Here's how the part is built. I have some questions about the finished solid (model axes, mm). A direction names the side the tool comes from. Coordinates: 2 decimals unless noted, no trailing zeros. Write each loop counter-clockwise with the first axis right and the second up, starting at its lowest first coordinate (ties: lowest second). Pieces come first, ordered by that corner, then holes.
Item 1: For faces 1 (the face through (-10.662, -17, 3)), 2 (the face through (-0.515, -38.635, 0.601)), which set-ups out of +Z, -Z, +X, -X, +Y, -Y let a thin tool reach every point of the face, with its end or its side?
Item 2: If we section it at A-A (z = 3.9): Please give me the cut outline in (x, y), then the cut area to 3 significant figures.
Item 3: If we section it at B-B (x = 8.75): Please give me the cut outline in (y, z), then the cut area to 3 significant figures.
Item 4: I'm going to push a flat-ended pin straight in: pin 1 Ø5 at (x, y) = (3.5, -13) entering from +Z. Where does the tip first touch, or does it pass through?
Item 5: We'd pull the mould along X, two halves only. Please class faces 3 (the face through (-1, -36.706, 3)), 4 (the face through (-12.59, -16.42, 0.6)), 5 (the face through (-1, -39.206, 4)): +X half, -X half, draft (parallel to the pull), parting line (faces both ways), or undercut.
Item 6: If I drill on line 1 (Y direction, x = -3.5, z = 2.65); line 2 (X direction, y = -20, z = 3.55); line 3 (Z direction, x = -2.75, y = -17), over which ranges is the centre line in solid material (lowest first)?
Item 7: If we section it at C-C (y = -21.5): Please give me the cut outline in (x, z).
from build123d import *

# Parameters (mm, degrees)
IZIM1_W                     = 25
IZIM1_H                     = 45
Y_KSEKLIK_EKSTR_ZYON1_DEPTH = 5
IZIM2_W                     = 20
IZIM2_H                     = 40
KES_EKSTR_ZYON1_DEPTH       = 3.5
RADYUS1_R                   = 2


with BuildPart() as part:
    # Çizim1 → Yükseklik-Ekstrüzyon1 (new body)
    with BuildSketch(Plane.XY.offset(5)):
        with Locations((-0.661993769, -16.705607477)):
            Rectangle(IZIM1_W, IZIM1_H)
    extrude(amount=-Y_KSEKLIK_EKSTR_ZYON1_DEPTH)

    # Çizim2 → Kes-Ekstrüzyon1 (cut)
    with BuildSketch(Plane.XY.offset(5)):
        with Locations((-0.661993769, -16.705607477)):
            Rectangle(IZIM2_W, IZIM2_H)
    extrude(amount=-KES_EKSTR_ZYON1_DEPTH, mode=Mode.SUBTRACT)

    # Radyus1
    radyus1_edges = [part.edges().sort_by_distance(p)[0] for p in [
        (11.838006231, -16.705607477, 0),
        (-0.661993769, 5.794392523, 0),
        (-13.161993769, -16.705607477, 0),
        (-13.161993769, 5.794392523, 2.5),
        (11.838006231, 5.794392523, 2.5),
        (11.838006231, -39.205607477, 2.5),
        (-13.161993769, -39.205607477, 2.5),
        (-0.661993769, -39.205607477, 0),
    ]]
    fillet(radyus1_edges, radius=RADYUS1_R)


solid = part.part
Answer list:
1. face 1: +Z
1. face 2: -Z, +X, -X, -Y
2. outline: (-13.16, -37.21) arc R2 ccw to (-11.16, -39.21) - (9.84, -39.21) arc R2 ccw to (11.84, -37.21) - (11.84, 3.79) arc R2 ccw to (9.84, 5.79) - (-11.16, 5.79) arc R2 ccw to (-13.16, 3.79) - close; hole (-10.66, -36.71) - (9.34, -36.71) - (9.34, 3.29) - (-10.66, 3.29) - close
2. area: 322 mm2
3. outline: (-39.21, 2) arc R2 ccw to (-37.21, 0) - (3.79, 0) arc R2 ccw to (5.79, 2) - (5.79, 5) - (3.29, 5) - (3.29, 1.5) - (-36.71, 1.5) - (-36.71, 5) - (-39.21, 5) - close
3. area: 83.3 mm2
4. pin 1: stops at z = 1.5
5. face 3: undercut
5. face 4: -X half
5. face 5: draft
6. line 1: y = -39.21 to -36.71, 3.29 to 5.79
6. line 2: x = -13.16 to -10.66, 9.34 to 11.84
6. line 3: z = 0 to 1.5
7. outline: (-13.16, 2) arc R2 ccw to (-11.16, 0) - (9.84, 0) arc R2 ccw to (11.84, 2) - (11.84, 5) - (9.34, 5) - (9.34, 1.5) - (-10.66, 1.5) - (-10.66, 5) - (-13.16, 5) - close
